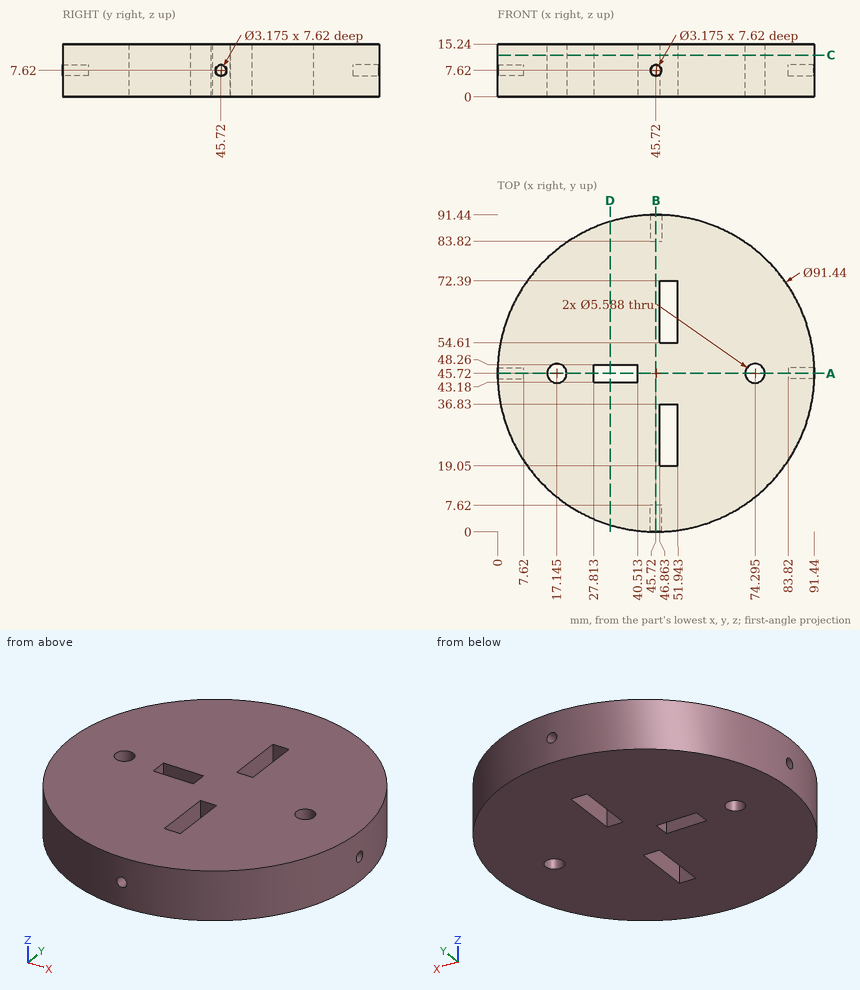
Check sheet for the drawn part. Datum: minimum x, y, z corner. Units: mm. Round coordinates to 2 decimals unless told otherwise and drop trailing zeros. Write each loop counter-clockwise with the first axis right and the second up, starting at its lowest first coordinate (ties: lowest second). Pieces come first, ordered by that corner, then holes. Notation, with made-up numbers: (80.5, 7) - (107.5, 7) arc R22 ccw to (107.5, 34) - close; hole circle Ø11 at (-31.75, 87.5). An arc over 180 degrees is marked (long way). Write each question's results on one line, items separated by ' | '.
(1) Depth check by flat-ended pin: pin 1 Ø2.5 at (y, z) = (45.72, 7.62) entering from -X; pin 2 Ø4.5 at (y, z) = (23.5, 8.5) entering from +X; pin 3 Ø1.5 at (x, z) = (76, 11.5) entering from -Y (1 decimal). Enter the tip coordinate at first touch or a pass-through.
Computed:
pin 1: stops at x = 7.62 | pin 2: stops at x = 86.85 | pin 3: stops at y = 10.8
(2) Sectioned sample at B-B, the plane x = 45.72. Enter the section's corners in (y, z), plus the area to 4 significant figures.
Computed:
outline: (0, 0) - (91.44, 0) - (91.44, 6.03) - (83.82, 6.03) - (83.82, 9.21) - (91.44, 9.21) - (91.44, 15.24) - (0, 15.24) - (0, 9.21) - (7.62, 9.21) - (7.62, 6.03) - (0, 6.03) - close | area: 1,345 mm^2
(3) Thickness scan on probe 1 along X at (y, z) = (46.5, 11.25); probe 2 along Y at (x, z) = (51.5, 10); probe 3 along Y at (x, z) = (15, 10.25). Record the ranges inside material, lowest first. Write a range as from..to.
Computed:
probe 1: x = 0.01..14.46, 19.83..27.81, 40.51..71.61, 76.98..91.43 | probe 2: y = 0.37..19.05, 36.83..54.61, 72.39..91.07 | probe 3: y = 11.86..43.93, 47.51..79.58
(4) Sectioned sample at A-A, the plane y = 45.72. Enter the section's corners in (x, z), plus the area to 3 significant figures.
Computed:
outline: (0, 0) - (14.35, 0) - (14.35, 15.24) - (0, 15.24) - (0, 9.21) - (7.62, 9.21) - (7.62, 6.03) - (0, 6.03) - close; (19.94, 0) - (27.81, 0) - (27.81, 15.24) - (19.94, 15.24) - close; (40.51, 0) - (71.5, 0) - (71.5, 15.24) - (40.51, 15.24) - close; (77.09, 0) - (91.44, 0) - (91.44, 6.03) - (83.82, 6.03) - (83.82, 9.21) - (91.44, 9.21) - (91.44, 15.24) - (77.09, 15.24) - close | area: 981 mm^2
(5) Sectioned sample at C-C, the plane z = 12. Count the separate pieces of the cut face and the enclosed holes in it, plus the area to 3 significant figures.
Computed:
separate pieces: 1 | enclosed holes: 5 | area: 6,270 mm^2
(6) Sectioned sample at D-D, the plane x = 32.5. Enter the section's corners in (y, z), plus the area to 3 significant figures.
Computed:
outline: (1.95, 0) - (43.18, 0) - (43.18, 15.24) - (1.95, 15.24) - close; (48.26, 0) - (89.49, 0) - (89.49, 15.24) - (48.26, 15.24) - close | area: 1,260 mm^2
